```python
from build123d import *

# Parameters (mm, degrees)
BOSS_EXTRUDE1_DEPTH = 28.575
SKETCH6_R           = 2.54
CUT_EXTRUDE4_DEPTH  = 28.575


with BuildPart() as part:
    # Sketch3 → Boss-Extrude1 (new body)
    with BuildSketch(Plane(origin=(0, 0, 0), x_dir=(1, 0, 0), z_dir=(0, 1, 0))):
        with BuildLine():
            Line((0, 0), (0, 0.635))
            ThreePointArc((0, 0.635), (-12.065, 12.7), (0, 24.765))
            Line((0, 24.765), (0, 25.4))
            Line((0, 25.4), (-25.4, 25.4))
            Line((-25.4, 25.4), (-25.4, 0))
            Line((-25.4, 0), (0, 0))
        make_face()
    extrude(amount=BOSS_EXTRUDE1_DEPTH)

    # Sketch6 → Cut-Extrude4 (cut)
    with BuildSketch(Plane(origin=(0, 0, 0), x_dir=(-1, 0, 0), z_dir=(0, -1, 0))):
        with Locations(Location((19.05, 12.7, 0), (0, 0, 90))):
            Circle(SKETCH6_R)
    extrude(amount=-CUT_EXTRUDE4_DEPTH, mode=Mode.SUBTRACT)


solid = part.part
```
Design review of the part built by this model. Coordinates are the model's own, in mm. Coordinates: 2 decimals unless noted, no trailing zeros. Loops run counter-clockwise (first coordinate to the right, second up) from the corner with the lowest first, then second, coordinate; pieces in that order, holes last. Notation, with made-up numbers: (-27, 37.5) - (32, 37.5) arc R22 cw to (32, 58.5) - close; hole circle Ø1 at (53, 74.25). An arc over 180 degrees is marked (long way). Use CSV: the item, a comma, the result in double quotes. Start each with the question number.
1) Wall thickness on L1, parallel to X at y = 11.75, z = -12.7 (3 decimals); L2, parallel to Z at x = -8.75, y = 26.5; L3, parallel to Z at x = -18, y = 22: over which ranges is each line inside the solid? List them lowest first. Write a range as from..to.
2) Consider section A-A on x = -19.05. Write out the cut boundary in (y, z) (3 decimals).
3) The part is to be moulded in two halves that separate along Z. For faces 1 (the flat face through (-13, 14, 0)), 2 (the cylindrical face through (-16.53, 14.09, -12.37)), 3 (the flat face through (-16, 28.575, -13)), say which applies: +Z half, -Z half, draft (parallel to the pull), parting line (faces both ways), or undercut.
4) For pin 1 Ø6 at (x, y) = (-14, 18) entering from +Z; pin 2 Ø8 at (y, z) = (17, -12.5) entering from +X, all flat-tipped, find the tip position at first contact; note any pin that passes through.
5) Consider section D-D on z = -7.5. Write out the cut boundary in (x, y) (3 decimals), then the cut area to 3 significant figures.
6) Consider section B-B on z = -12.7. Write out the cut boundary in (x, y) (3 decimals).
7) Consider section C-C on y = 9.75. Write out the cut boundary in (x, z) (3 decimals), then the cut area to 3 significant figures.
Geometry says:
1,L1,"-25.4..-21.59, -16.51..-12.065"
1,L2,"-25.4..-21.01, -4.39..0"
1,L3,"-25.4..-15.01, -10.39..0"
2,outline,"(0, -25.4) - (28.575, -25.4) - (28.575, -15.24) - (0, -15.24) - close; (0, -10.16) - (28.575, -10.16) - (28.575, 0) - (0, 0) - close"
3,face 1,"+Z half"
3,face 2,"undercut"
3,face 3,"draft"
4,pin 1,"z = 0"
4,pin 2,"x = -11.31"
5,outline,"(-25.4, 0) - (-10.887, 0) - (-10.887, 28.575) - (-25.4, 28.575) - close"
5,area,"415 mm^2"
6,outline,"(-25.4, 0) - (-21.59, 0) - (-21.59, 28.575) - (-25.4, 28.575) - close; (-16.51, 0) - (-12.065, 0) - (-12.065, 28.575) - (-16.51, 28.575) - close"
7,outline,"(-25.4, -25.4) - (0, -25.4) - (0, -24.765) arc R12.065 cw to (0, -0.635) - (0, 0) - (-25.4, 0) - close; hole circle Ø5.08 at (-19.05, -12.7)"
7,area,"396 mm^2"
